Read the model definition and answer for the solid it produces. Units are mm, in the model's axes. Coordinates: 2 decimals unless noted, no trailing zeros. Write each loop counter-clockwise with the first axis right and the second up, starting at its lowest first coordinate (ties: lowest second). Pieces come first, ordered by that corner, then holes.
(1) Section C-C on y = -96 is taken. Write down the section's boundary in (x, z), then the cut area to 3 significant figures.
(2) The mould has two halves that part along Y. Classify faces 1 (the flat face through (-1, 0, 1)), 2 (the cylindrical face through (2.75, -67.7, -0.52)), 3 (the flat face through (-14, -58, -37.331)), 4 (the flat face through (-35, -117.227, 1)): +Y half, -Y half, draft (parallel to the pull), parting line (faces both ways), or undercut.
(3) Given pin 1 (3 mm diameter, centred on y = -76.5, z = -18.5, fed in from +X); pin 2 (23 mm diameter, centred on x = 0, y = -55.3, fed in from +Z), each flat-ended and moving along its own axis, determine where each tip first touches the part or whether it passes through.
(4) Find the intervals of material crossed by probe 1 along Y at (x, z) = (2.5, 7); probe 2 along Y at (x, z) = (6.5, -25); probe 3 along X at (y, z) = (-52.5, 18.5), in increasing order.
(5) Section A-A on x = 0 is taken. Write down the section's boundary in (y, z), then the cut area to 3 significant figures.
(6) Section B-B on z = -24.5 is taken. Write down the section's boundary in (x, y), then the cut area to 3 significant figures.
(7) Section D-D on x = 44 is taken. Write down the section's boundary in (y, z), then the cut area to 3 significant figures.
from build123d import *

# Parameters (mm, degrees)
F0_W     = 121.796116
F0_H     = 74.661746
F1_DEPTH = 117.227465
F3_D     = 25.4
F4_R     = 69.925974


with BuildPart() as f1:
    # F0 (on Front) → F1 (new body)
    with BuildSketch(Plane.XZ):
        Rectangle(F0_W, F0_H)
    extrude(amount=F1_DEPTH)

    # F3 (through all)
    with Locations(Plane.XY.offset(37.330873)):
        with Locations((0, -55.301771)):
            Hole(F3_D / 2)

    # F4
    f4_edges = [f1.edges().sort_by_distance(p)[0] for p in [
        (60.898058, -117.227465, 0),
    ]]
    fillet(f4_edges, radius=F4_R)


solid = f1.part
Response:
1. outline: (-60.9, -37.33) - (41.15, -37.33) - (41.15, 37.33) - (-60.9, 37.33) - close
1. area: 7,620 mm2
2. face 1: +Y half
2. face 2: undercut
2. face 3: draft
2. face 4: -Y half
3. pin 1: stops at x = 55.18
3. pin 2: passes through
4. probe 1: y = -116.27 to -67.75, -42.85 to 0
4. probe 2: y = -115.48 to -66.21, -44.39 to 0
4. probe 3: x = -60.9 to -12.39, 12.39 to 60.7
5. outline: (-116.64, -37.33) - (-68, -37.33) - (-68, 37.33) - (-116.64, 37.33) - close; (-42.6, -37.33) - (0, -37.33) - (0, 37.33) - (-42.6, 37.33) - close
5. area: 6,810 mm2
6. outline: (-60.9, -117.23) - (-9.03, -117.23) arc R69.93 ccw to (60.9, -47.3) - (60.9, 0) - (-60.9, 0) - close; hole circle Ø25.4 at (0, -55.3)
6. area: 12,700 mm2
7. outline: (-92.88, -37.33) - (0, -37.33) - (0, 37.33) - (-92.88, 37.33) - close
7. area: 6,930 mm2
